Design review of the part shown in the three views and the two pictorial views. Dimensions are in mm from the part's minimum x, y and z. Round coordinates to 2 decimals unless told otherwise and drop trailing zeros. Loops run counter-clockwise (first coordinate to the right, second up) from the corner with the lowest first, then second, coordinate; pieces in that order, holes last.
1. Consider section B-B on y = 18.5. State the section outline as (x, z) points (1 decimal).
2. Consider section A-A on x = 0.6. State the section outline as (y, z) points (1 decimal), then the cut area to 3 significant figures.
3. Draft analysis for pull direction Z (two halves, no side actions). For the marked faces 1, 2, 3 and 4, state which applies: released by +Z, released by -Z, zero draft, split by the parting line, or undercut.
4. Consider section D-D on y = 13.5. State the section outline as (x, z) points (1 decimal).
5. To check wall thickness, follow line 1 along Z through (x, y) = (2.05, 28.5); line 2 along Y through (x, z) = (0.4, 29) (1 decimal); line 3 along Y through (x, z) = (1.5, 25.5) (1 decimal). State the ranges of each line that lie inside material, in increasing order.
6. Clearance check with flat-ended pins moving along their axes: pin 1 Ø2 at (y, z) = (10.5, 46.5) entering from -X; pin 2 Ø1.6 at (x, y) = (2, 25.5) entering from +Z; pin 3 Ø1 at (x, y) = (1, 26) entering from -Z; pin 4 Ø1.6 at (x, y) = (1, 28.5) entering from -Z. State where each tip first meets the part, or that it passes through.
7. Consider section C-C on z = 26. State the section outline as (x, y) points (1 decimal).
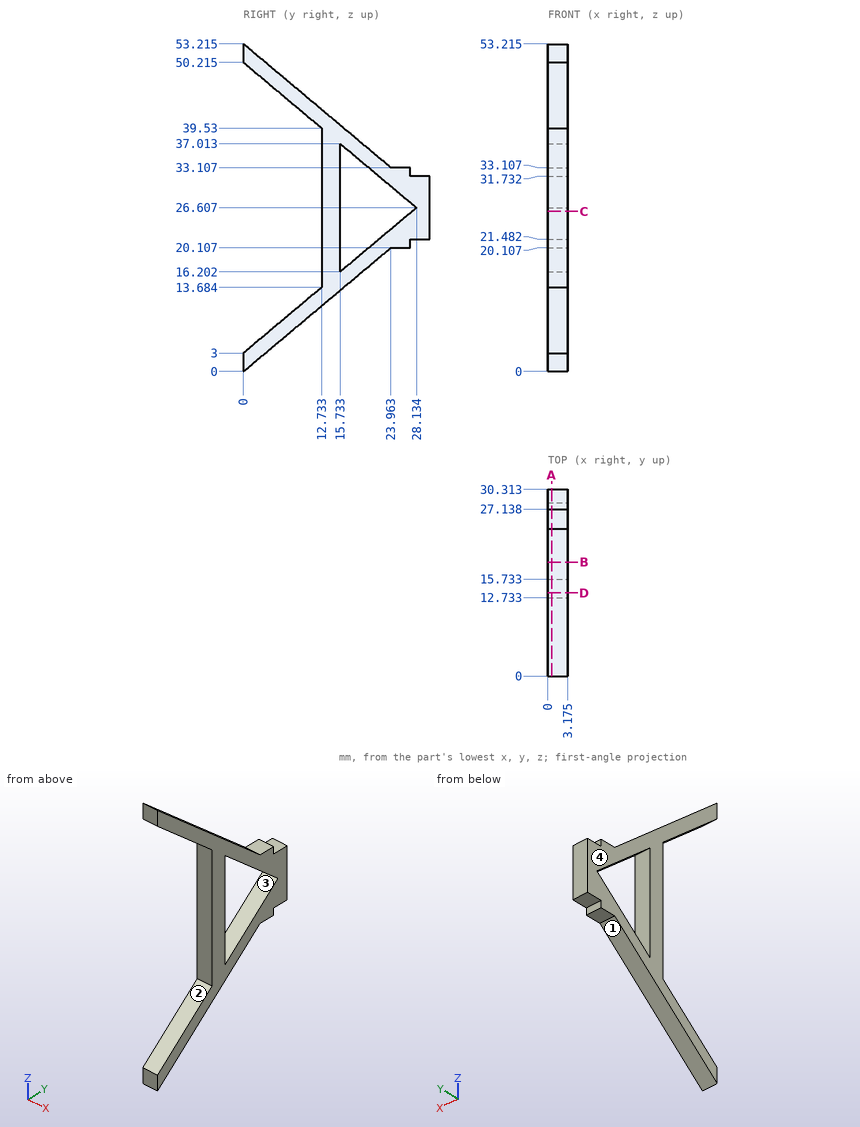
Resolved:
1. outline: (0, 15.5) - (3.2, 15.5) - (3.2, 18.5) - (0, 18.5) - close; (0, 34.7) - (3.2, 34.7) - (3.2, 37.7) - (0, 37.7) - close
2. outline: (0, 0) - (24, 20.1) - (27.1, 20.1) - (27.1, 21.5) - (30.3, 21.5) - (30.3, 31.7) - (27.1, 31.7) - (27.1, 33.1) - (24, 33.1) - (0, 53.2) - (0, 50.2) - (12.7, 39.5) - (12.7, 13.7) - (0, 3) - close; hole (15.7, 16.2) - (28.1, 26.6) - (15.7, 37) - close
2. area: 273 mm2
3. face 1: released by -Z
3. face 2: undercut
3. face 3: undercut
3. face 4: zero draft
4. outline: (0, 11.3) - (3.2, 11.3) - (3.2, 41.9) - (0, 41.9) - close
5. line 1: z = 21.48 to 31.73
5. line 2: y = 12.7 to 15.7, 25.3 to 30.3
5. line 3: y = 12.7 to 15.7, 26.8 to 30.3
6. pin 1: passes through
6. pin 2: stops at z = 33.11
6. pin 3: stops at z = 20.11
6. pin 4: stops at z = 21.48
7. outline: (0, 12.7) - (3.2, 12.7) - (3.2, 15.7) - (0, 15.7) - close; (0, 27.4) - (3.2, 27.4) - (3.2, 30.3) - (0, 30.3) - close
